Design review of the part built by this model. Coordinates are the model's own, in mm. A direction names the side the tool comes from. Round coordinates to 2 decimals unless told otherwise and drop trailing zeros. Order: outer loops, then holes, each group sorted by start corner. A loop starts at its lowest first (then second) coordinate and runs counter-clockwise, first axis right, second up. Notation, with made-up numbers: (9.5, 12) - (53.5, 12) arc R14 ccw to (53.5, 16) - close; hole circle Ø2 at (55.5, 62). An arc over 180 degrees is marked (long way). Write item = value, one per line.
from build123d import *

# Parameters (mm, degrees)
F0_W     = 15
F0_H     = 12
F1_DEPTH = 2.625
F2_W     = 2
F2_H     = 4
F3_DEPTH = 3.05
F4_R     = 0.4
F5_DEPTH = 25
F6_R     = 0.99999
F7_R     = 1
F8_DEPTH = 25


# Not quite as in the source:
# - a fillet or chamfer is up to 0.001 mm smaller than in the source, because OpenCascade refuses the exact size


with BuildPart() as f1:
    # F0 (on Front) → F1 (new body)
    with BuildSketch(Plane.XZ):
        Rectangle(F0_W, F0_H)
    extrude(amount=F1_DEPTH)

    # F2 (on face) → F3 (join)
    with BuildSketch(Plane.XZ.offset(2.625)):
        with Locations((6.5, 4)):
            Rectangle(F2_W, F2_H)
        with Locations((6.5, -4)):
            Rectangle(F2_W, F2_H)
    extrude(amount=F3_DEPTH)

    # F4 (on face) → F5 (cut)
    with BuildSketch(Plane(origin=(0, 0, -6), x_dir=(1, 0, 0), z_dir=(0, 0, -1))):
        with Locations((6.5, 4.15)):
            Circle(F4_R)
    extrude(amount=-F5_DEPTH, mode=Mode.SUBTRACT)

    # F6 (radius 1 in the source; OpenCascade refuses exactly that, so slightly less here)
    f6_edges = [f1.edges().sort_by_distance(p)[0] for p in [
        (7.5, -5.675, 4),
        (5.5, -5.675, 4),
        (7.5, -5.675, -4),
        (5.5, -5.675, -4),
    ]]
    fillet(f6_edges, radius=F6_R)

    # F7 (on face) → F8 (cut)
    with BuildSketch(Plane(origin=(0, 0, 0), x_dir=(-1, 0, 0), z_dir=(0, 1, 0))):
        with Locations((0, 3.5)):
            Circle(F7_R)
        with Locations((0, -3.5)):
            Circle(F7_R)
    extrude(amount=-F8_DEPTH, mode=Mode.SUBTRACT)


solid = f1.part
Item 1: The part is to be moulded in two halves that separate along Z. For faces 1 (the face through (0, -2, -6)), 2 (the face through (6.93, -3.79, -2)), 3 (the face through (6.41, -3.76, 3.97)), say which applies: +Z half, -Z half, draft (parallel to the pull), parting line (faces both ways), or undercut.
Data:
face_1 = -Z half
face_2 = undercut
face_3 = draft
Item 2: Insertion check: P1, Ø6, axis at x = 1.5, z = -2, coming from the -Y side (3 decimals); P2, Ø1, axis at y = -4, z = -5, coming from the -X side. Each pin has a flat end and moves straight along its axis. Give the tip position at first contact, or say it passes through.
Data:
P1 = -2.625
P2 = 5.5
Item 3: Take a section at B-B, the plane y = -4.15. State the section outline as (x, z) points.
Data:
outline = (5.5, -6) - (6.1, -6) - (6.1, -2) - (5.5, -2) - close; (5.5, 2) - (6.1, 2) - (6.1, 6) - (5.5, 6) - close; (6.9, -6) - (7.5, -6) - (7.5, -2) - (6.9, -2) - close; (6.9, 2) - (7.5, 2) - (7.5, 6) - (6.9, 6) - close
Item 4: For faces 4 (the face through (-7.5, -1, 0)), 5 (the face through (5.5, -4, 4)), 6 (the face through (6.93, -3.79, 2)), list the 3-axis set-ups (+Z, -Z, +X, -X, +Y, -Y) from which the entire face can be reached by the end or side of a thin tool; tool diameter is ignored.
Data:
face_4 = +Z, -Z, -X, +Y, -Y
face_5 = +Z, -Z, -X, -Y
face_6 = +X, -X, -Y
Item 5: For line 1 along Z through (x, y) = (0, -1.7); line 2 along X through (y, z) = (-4.15, -4.25); line 3 along Y through (x, z) = (6.5, 3.05) (3 decimals), list the stretches that pass through material, from the lowest coordinate up. Write a range as [from, to].
Data:
line_1 = [-6, -4.5], [-2.5, 2.5], [4.5, 6]
line_2 = [5.5, 6.1], [6.9, 7.5]
line_3 = [-5.675, -4.55], [-3.75, 0]
Item 6: Take a section at C-C, the plane y = -2.9. State the section outline as (x, z) points, and give its area (3 significant figures).
Data:
outline = (5.5, -6) - (7.5, -6) - (7.5, -2) - (5.5, -2) - close; (5.5, 2) - (7.5, 2) - (7.5, 6) - (5.5, 6) - close
area = 16.0 mm2
Item 7: Take a section at D-D, the plane x = 0. State the section outline as (y, z) points (3 decimals).
Data:
outline = (-2.625, -6) - (0, -6) - (0, -4.5) - (-2.625, -4.5) - close; (-2.625, -2.5) - (0, -2.5) - (0, 2.5) - (-2.625, 2.5) - close; (-2.625, 4.5) - (0, 4.5) - (0, 6) - (-2.625, 6) - close
Item 8: Take a section at A-A, the plane z = -3.5. Count the separate pieces of the cut face and the enclosed holes in it, and give its area (3 significant figures).
Data:
separate_pieces = 2
enclosed_holes = 1
area = 39.3 mm2
